Work out the finished part from the listing and answer in its coordinate system (mm). Face numbers are marked on the shaded views. A direction names the side the tool comes from. Give positions to 0.01 mm unless a question says otherwise; leave off trailing zeros. Write each loop counter-clockwise with the first axis right and the second up, starting at its lowest first coordinate (ties: lowest second). Pieces come first, ordered by that corner, then holes. Notation, with made-up numbers: (70.5, 88.25) - (108.5, 88.25) arc R20 cw to (108.5, 101.25) - close; hole circle Ø10 at (84, -14). An arc over 180 degrees is marked (long way). Write item = value, one per line.
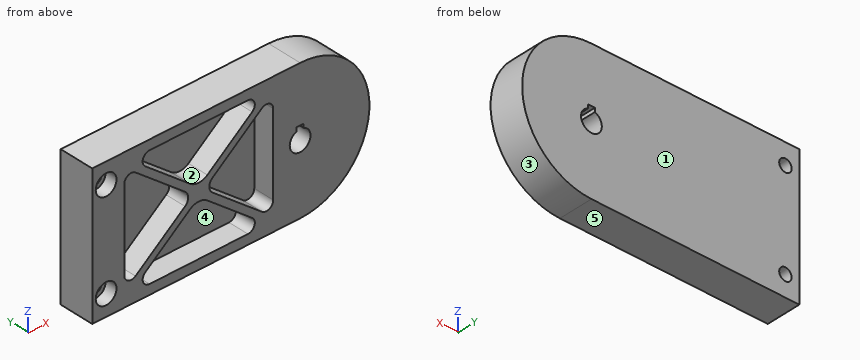
from build123d import *

# Parameters (mm, degrees)
DODANIE_WYCI_GNI_CIE1_DEPTH                         = 25
POG_BIENIE_WALCOWE_POD_M8_WKR_T_Z_BEM_W_D           = 9
POG_BIENIE_WALCOWE_POD_M8_WKR_T_Z_BEM_W_DEPTH       = 26.25
POG_BIENIE_WALCOWE_POD_M8_WKR_T_Z_BEM_W_CBORE_D     = 15
POG_BIENIE_WALCOWE_POD_M8_WKR_T_Z_BEM_W_CBORE_DEPTH = 8.6
POG_BIENIE_WALCOWE_POD_M8_WKR_T_Z_BEM_W_TIP         = 2.703872786
WYTNIJ_WYCI_GNI_CIE1_DEPTH                          = 15


with BuildPart() as part:
    # Szkic1 → Dodanie-wyciągnięcie1 (new body)
    with BuildSketch(Plane(origin=(0, 0, 0), x_dir=(1, 0, 0), z_dir=(0, 1, 0))):
        with BuildLine():
            Line((0, -50), (0, 50))
            Line((0, 50), (150, 50))
            ThreePointArc((150, 50), (200, 0), (150, -50))
            Line((150, -50), (0, -50))
        make_face()
        with BuildLine():
            Line((147.5, -9.8), (152.5, -9.8))
            Line((152.5, -9.8), (152.5, -7.071067812))
            ThreePointArc((152.5, -7.071067812), (150, 7.5), (147.5, -7.071067812))
            Line((147.5, -7.071067812), (147.5, -9.8))
        make_face(mode=Mode.SUBTRACT)
    extrude(amount=DODANIE_WYCI_GNI_CIE1_DEPTH)

    # Pogłębienie walcowe pod M8 Wkręt z łbem walcowym z gniazdem sześciokątnym1
    with Locations(Plane(origin=(10, 0, 35), x_dir=(0, 0, -1), z_dir=(0, -1, 0))):
        with Locations((0, 0), (70, 0)):
            CounterBoreHole(POG_BIENIE_WALCOWE_POD_M8_WKR_T_Z_BEM_W_D / 2, POG_BIENIE_WALCOWE_POD_M8_WKR_T_Z_BEM_W_CBORE_D / 2, POG_BIENIE_WALCOWE_POD_M8_WKR_T_Z_BEM_W_CBORE_DEPTH, depth=POG_BIENIE_WALCOWE_POD_M8_WKR_T_Z_BEM_W_DEPTH)
            with Locations((0, 0, -(POG_BIENIE_WALCOWE_POD_M8_WKR_T_Z_BEM_W_DEPTH + POG_BIENIE_WALCOWE_POD_M8_WKR_T_Z_BEM_W_TIP / 2))):  # 118° drill point
                Cone(0, POG_BIENIE_WALCOWE_POD_M8_WKR_T_Z_BEM_W_D / 2, POG_BIENIE_WALCOWE_POD_M8_WKR_T_Z_BEM_W_TIP, mode=Mode.SUBTRACT)

    # Szkic4 → Wytnij-wyciągnięcie1 (cut)
    with BuildSketch(Plane.XZ):
        with BuildLine():
            Line((31.213273393, 33.297016557), (66.968494236, 4.684692061))
            ThreePointArc((66.968494236, 4.684692061), (69.219673049, 0), (66.968494236, -4.684692061))
            Line((66.968494236, -4.684692061), (31.213273393, -33.297016557))
            ThreePointArc((31.213273393, -33.297016557), (25.923625146, -33.899773139), (23.089255738, -29.393106506))
            Line((23.089255738, -29.393106506), (23.089255738, 29.393106506))
            ThreePointArc((23.089255738, 29.393106506), (25.923625146, 33.899773139), (31.213273393, 33.297016557))
        make_face()
        with BuildLine():
            Line((41.341249338, -43), (112.306649775, -43))
            ThreePointArc((112.306649775, -43), (117.024676389, -39.655362459), (115.430667431, -34.096089949))
            Line((115.430667431, -34.096089949), (83.071984868, -8.201770072))
            ThreePointArc((83.071984868, -8.201770072), (76.823949557, -6.009590175), (70.575914246, -8.201770072))
            Line((70.575914246, -8.201770072), (38.217231683, -34.096089949))
            ThreePointArc((38.217231683, -34.096089949), (36.623222725, -39.655362459), (41.341249338, -43))
        make_face()
        with BuildLine():
            Line((130.558643376, -29.393106506), (130.558643376, 29.393106506))
            ThreePointArc((130.558643376, 29.393106506), (127.724273968, 33.899773139), (122.43462572, 33.297016557))
            Line((122.43462572, 33.297016557), (86.679404878, 4.684692061))
            ThreePointArc((86.679404878, 4.684692061), (84.428226064, 0), (86.679404878, -4.684692061))
            Line((86.679404878, -4.684692061), (122.43462572, -33.297016557))
            ThreePointArc((122.43462572, -33.297016557), (127.724273968, -33.899773139), (130.558643376, -29.393106506))
        make_face()
        with BuildLine():
            Line((41.341249338, 43), (112.306649775, 43))
            ThreePointArc((112.306649775, 43), (117.024676389, 39.655362459), (115.430667431, 34.096089949))
            Line((115.430667431, 34.096089949), (83.071984868, 8.201770072))
            ThreePointArc((83.071984868, 8.201770072), (76.823949557, 6.009590175), (70.575914246, 8.201770072))
            Line((70.575914246, 8.201770072), (38.217231683, 34.096089949))
            ThreePointArc((38.217231683, 34.096089949), (36.623222725, 39.655362459), (41.341249338, 43))
        make_face()
    extrude(amount=-WYTNIJ_WYCI_GNI_CIE1_DEPTH, mode=Mode.SUBTRACT)


solid = part.part
1. Given pin 1 (0.8 mm diameter, centred on y = 15.5, z = 8.5, fed in from +X); pin 2 (5 mm diameter, centred on y = 22.5, z = 24, fed in from +X); pin 3 (10 mm diameter, centred on x = 61, z = -32, fed in from -Y), each flat-ended and moving along its own axis, determine where each tip first touches the part or whether it passes through.
Solution:
pin_1 = 199.34
pin_2 = 195.14
pin_3 = 15
2. For a pull along X with two mould halves and no side action, classify the marked faces 3, 4 and 5 as pulls with the +X half, pulls with the -X half, needs draft (parallel to the pull), parting line crosses it, or undercut.
Solution:
face_3 = pulls with the +X half
face_4 = undercut
face_5 = needs draft
3. Find section A-A, the plane y = 6.25. Give the number of separate pieces and of enclosed holes in the cut face, then the cut area to 3 significant figures.
Solution:
separate_pieces = 1
enclosed_holes = 7
area = 10,800 mm^2
4. Straight lines are drawn through the part: line 1 (Z direction, x = 101.5, y = 5.75); line 2 (X direction, y = 12.5, z = 28.5); line 3 (X direction, y = 10, z = -17). For each, find the intervals that lie inside material, in ascending order.
Solution:
line_1 = -50 to -43, -22.95 to -16.54, 16.54 to 22.95, 43 to 50
line_2 = 0 to 23.09, 37.21 to 45.21, 108.44 to 116.44, 130.56 to 191.08
line_3 = 0 to 23.09, 51.58 to 59.58, 94.07 to 102.07, 130.56 to 197.02
5. Find section D-D, the plane x = 59. Give the vertices of the cut face in (y, z), then the cut area to 3 significant figures.
Solution:
outline = (0, -50) - (25, -50) - (25, 50) - (0, 50) - (0, 43) - (15, 43) - (15, 17.47) - (0, 17.47) - (0, 11.06) - (15, 11.06) - (15, -11.06) - (0, -11.06) - (0, -17.47) - (15, -17.47) - (15, -43) - (0, -43) - close
area = 1,400 mm^2
6. Find section B-B, the plane z = 0. Give the vertices of the cut face in (x, y), then the cut area to 3 significant figures.
Solution:
outline = (0, 0) - (23.09, 0) - (23.09, 15) - (69.22, 15) - (69.22, 0) - (84.43, 0) - (84.43, 15) - (130.56, 15) - (130.56, 0) - (142.5, 0) - (142.5, 25) - (0, 25) - close; (157.5, 0) - (200, 0) - (200, 25) - (157.5, 25) - close
area = 3,240 mm^2
7. Find section C-C, the plane x = 10. Give the vertices of the cut face in (y, z).
Solution:
outline = (0, -50) - (25, -50) - (25, -39.5) - (8.6, -39.5) - (8.6, -42.5) - (0, -42.5) - close; (0, -27.5) - (8.6, -27.5) - (8.6, -30.5) - (25, -30.5) - (25, 30.5) - (8.6, 30.5) - (8.6, 27.5) - (0, 27.5) - close; (0, 42.5) - (8.6, 42.5) - (8.6, 39.5) - (25, 39.5) - (25, 50) - (0, 50) - close
8. A tool of negligible diameter and unlimited length cuts with its end or side. For the marked faces 1 and 2, from which of +Z, -Z, +X, -X, +Y, -Y can it reach the whole face along a straight path? Write none if from no direction.
Solution:
face_1 = +Z, -Z, +X, -X, +Y
face_2 = -Y
